Answer from the drawing. Dimensions are ordinates in mm from the lowest x, y and z of the part. Coordinates: 2 decimals unless noted, no trailing zeros. Write each loop counter-clockwise with the first axis right and the second up, starting at its lowest first coordinate (ties: lowest second). Pieces come first, ordered by that corner, then holes. Notation, with made-up numbers: (55, 77.5) - (91, 77.5) arc R25 ccw to (91, 89.5) - close; hole circle Ø3 at (-10.5, -18). An arc over 180 degrees is marked (long way). Return JSON: item names as keys, results as strings.
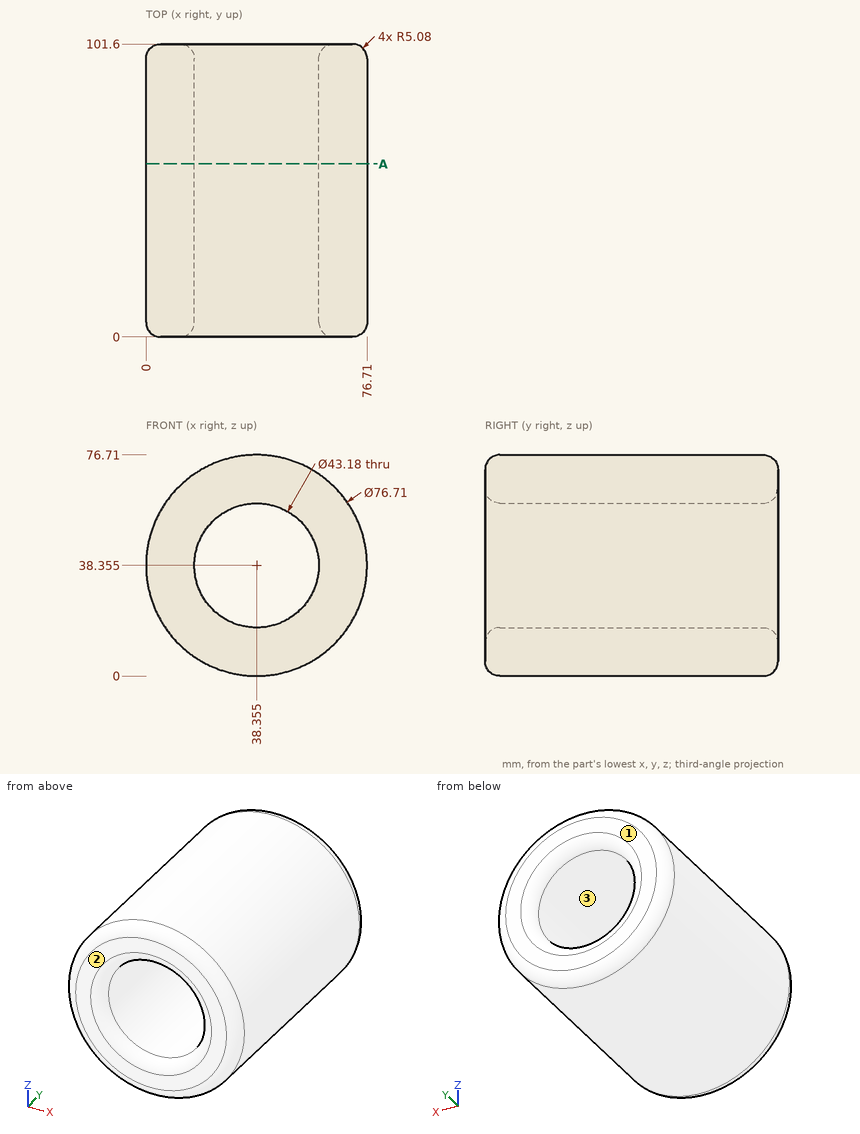
(1) Flat-ended cylindrical pins translate along their axes: P1, Ø12, axis at y = 47.5, z = 23, coming from the +X side; P2, Ø2, axis at x = 54.5, y = 14.5, coming from the +Z side; P3, Ø12, axis at y = 26.5, z = 22.5, coming from the -X side. Find the tip coordinate at first contact, or state that the pin passes through.
Answer:
{"P1": "x = 75.55", "P2": "z = 73.59", "P3": "x = 1.29"}
(2) Straight lines are drawn through the part: line 1 (X direction, y = 76, z = 24.5); line 2 (X direction, y = 89.5, z = 36.5) (1 decimal); line 3 (Z direction, x = 25, y = 31). For each, find the intervals that lie inside material, in ascending order. Write a range as from..to.
Answer:
{"line 1": "2.59..21.8, 54.91..74.12", "line 2": "0..16.8, 59.9..76.7", "line 3": "2.4..21.39, 55.32..74.31"}
(3) A cutting plane is placed at A-A (y = 60). Determine the outline of the cut face in (x, z) (3 decimals).
Answer:
{"outline": "circle Ø76.71 at (38.355, 38.355); hole circle Ø43.18 at (38.355, 38.355)"}
(4) Determine the mould class of the marked faces 1, 2 and 3 for opening direction Y: +Y half, -Y half, draft (parallel to the pull), parting line (faces both ways), or undercut.
Answer:
{"face 1": "+Y half", "face 2": "-Y half", "face 3": "draft"}
